```python
from build123d import *

# Parameters (mm, degrees)
F1_DEPTH = 45
F3_DEPTH = 45
F4_R     = 1.1
F5_DEPTH = 45
F6_R     = 3
F7_DEPTH = 0.1
F8_R     = 2.5
F9_DEPTH = 3


with BuildPart() as f1:
    # F0 (on Top) → F1 (new body)
    with BuildSketch(Plane.XY):
        with BuildLine():
            ThreePointArc((4.8636480497, -1.1597101572), (4.9657950143, -0.5838491892), (5, 0))
            ThreePointArc((5, 0), (4.9657950143, 0.5838491892), (4.8636480497, 1.1597101572))
            Line((4.8636480497, 1.1597101572), (1.294427191, 0))
            Line((1.294427191, 0), (4.8636480497, -1.1597101572))
        make_face()
        with BuildLine():
            Line((1.294427191, 0), (4.8636480497, 1.1597101572))
            ThreePointArc((4.8636480497, 1.1597101572), (4.7552825815, 1.5450849719), (4.6164344542, 1.9205553702))
            Line((4.6164344542, 1.9205553702), (1.0472135955, 0.760845213))
            Line((1.0472135955, 0.760845213), (0.6472135955, 0.2102924448))
            Line((0.6472135955, 0.2102924448), (1.294427191, 0))
        make_face()
        with BuildLine():
            ThreePointArc((4.6164344542, 1.9205553702), (4.7552825815, 1.5450849719), (4.8636480497, 1.1597101572))
            Line((4.8636480497, 1.1597101572), (67.6486194547, 21.5597839941))
            Line((67.6486194547, 21.5597839941), (67.4014058592, 22.3206292071))
            Line((67.4014058592, 22.3206292071), (4.6164344542, 1.9205553702))
        make_face()
        with BuildLine():
            Line((67.6486194547, -21.5597839941), (4.8636480497, -1.1597101572))
            ThreePointArc((4.8636480497, -1.1597101572), (4.7552825815, -1.5450849719), (4.6164344542, -1.9205553702))
            Line((4.6164344542, -1.9205553702), (67.4014058592, -22.3206292071))
            Line((67.4014058592, -22.3206292071), (67.6486194547, -21.5597839941))
        make_face()
        with BuildLine():
            ThreePointArc((4.6164344542, -1.9205553702), (4.7552825815, -1.5450849719), (4.8636480497, -1.1597101572))
            Line((4.8636480497, -1.1597101572), (1.294427191, 0))
            Line((1.294427191, 0), (0.6472135955, -0.2102924448))
            Line((0.6472135955, -0.2102924448), (1.0472135955, -0.760845213))
            Line((1.0472135955, -0.760845213), (4.6164344542, -1.9205553702))
        make_face()
        with BuildLine():
            Line((1.0472135955, 0.760845213), (4.6164344542, 1.9205553702))
            ThreePointArc((4.6164344542, 1.9205553702), (4.0450849719, 2.9389262615), (3.2531133995, 3.7970058217))
            Line((3.2531133995, 3.7970058217), (1.0472135955, 0.760845213))
        make_face()
        with BuildLine():
            ThreePointArc((3.2531133995, -3.7970058217), (4.0450849719, -2.9389262615), (4.6164344542, -1.9205553702))
            Line((4.6164344542, -1.9205553702), (1.0472135955, -0.760845213))
            Line((1.0472135955, -0.760845213), (3.2531133995, -3.7970058217))
        make_face()
        with BuildLine():
            Line((1.0472135955, 0.760845213), (3.2531133995, 3.7970058217))
            ThreePointArc((3.2531133995, 3.7970058217), (2.9389262615, 4.0450849719), (2.605899804, 4.2672340235))
            Line((2.605899804, 4.2672340235), (0.4, 1.2310734149))
            Line((0.4, 1.2310734149), (0.4, 0.5505527682))
            Line((0.4, 0.5505527682), (1.0472135955, 0.760845213))
        make_face()
        with BuildLine():
            ThreePointArc((2.605899804, 4.2672340235), (2.9389262615, 4.0450849719), (3.2531133995, 3.7970058217))
            Line((3.2531133995, 3.7970058217), (42.0563597105, 57.2050924997))
            Line((42.0563597105, 57.2050924997), (41.409146115, 57.6753207015))
            Line((41.409146115, 57.6753207015), (2.605899804, 4.2672340235))
        make_face()
        with BuildLine():
            Line((42.0563597105, -57.2050924997), (3.2531133995, -3.7970058217))
            ThreePointArc((3.2531133995, -3.7970058217), (2.9389262615, -4.0450849719), (2.605899804, -4.2672340235))
            Line((2.605899804, -4.2672340235), (41.409146115, -57.6753207015))
            Line((41.409146115, -57.6753207015), (42.0563597105, -57.2050924997))
        make_face()
        with BuildLine():
            ThreePointArc((2.605899804, -4.2672340235), (2.9389262615, -4.0450849719), (3.2531133995, -3.7970058217))
            Line((3.2531133995, -3.7970058217), (1.0472135955, -0.760845213))
            Line((1.0472135955, -0.760845213), (0.4, -0.5505527682))
            Line((0.4, -0.5505527682), (0.4, -1.2310734149))
            Line((0.4, -1.2310734149), (2.605899804, -4.2672340235))
        make_face()
        with BuildLine():
            Line((0.4, 1.2310734149), (2.605899804, 4.2672340235))
            ThreePointArc((2.605899804, 4.2672340235), (1.5450849719, 4.7552825815), (0.4, 4.9839743178))
            Line((0.4, 4.9839743178), (0.4, 1.2310734149))
        make_face()
        with BuildLine():
            ThreePointArc((0.4, -4.9839743178), (1.5450849719, -4.7552825815), (2.605899804, -4.2672340235))
            Line((2.605899804, -4.2672340235), (0.4, -1.2310734149))
            Line((0.4, -1.2310734149), (0.4, -4.9839743178))
        make_face()
        with BuildLine():
            Line((0.4, 1.2310734149), (0.4, 4.9839743178))
            ThreePointArc((0.4, 4.9839743178), (0, 5), (-0.4, 4.9839743178))
            Line((-0.4, 4.9839743178), (-0.4, 1.2310734149))
            Line((-0.4, 1.2310734149), (0, 0.6805206467))
            Line((0, 0.6805206467), (0.4, 1.2310734149))
        make_face()
        with BuildLine():
            ThreePointArc((-0.4, 4.9839743178), (0, 5), (0.4, 4.9839743178))
            Line((0.4, 4.9839743178), (0.4, 71))
            Line((0.4, 71), (-0.4, 71))
            Line((-0.4, 71), (-0.4, 4.9839743178))
        make_face()
        with BuildLine():
            Line((0.4, -71), (0.4, -4.9839743178))
            ThreePointArc((0.4, -4.9839743178), (0, -5), (-0.4, -4.9839743178))
            Line((-0.4, -4.9839743178), (-0.4, -71))
            Line((-0.4, -71), (0.4, -71))
        make_face()
        with BuildLine():
            ThreePointArc((-0.4, -4.9839743178), (0, -5), (0.4, -4.9839743178))
            Line((0.4, -4.9839743178), (0.4, -1.2310734149))
            Line((0.4, -1.2310734149), (0, -0.6805206467))
            Line((0, -0.6805206467), (-0.4, -1.2310734149))
            Line((-0.4, -1.2310734149), (-0.4, -4.9839743178))
        make_face()
        with BuildLine():
            Line((-0.4, 1.2310734149), (-0.4, 4.9839743178))
            ThreePointArc((-0.4, 4.9839743178), (-1.5450849719, 4.7552825815), (-2.605899804, 4.2672340235))
            Line((-2.605899804, 4.2672340235), (-0.4, 1.2310734149))
        make_face()
        with BuildLine():
            ThreePointArc((-2.605899804, -4.2672340235), (-1.5450849719, -4.7552825815), (-0.4, -4.9839743178))
            Line((-0.4, -4.9839743178), (-0.4, -1.2310734149))
            Line((-0.4, -1.2310734149), (-2.605899804, -4.2672340235))
        make_face()
        with BuildLine():
            Line((-0.4, 1.2310734149), (-2.605899804, 4.2672340235))
            ThreePointArc((-2.605899804, 4.2672340235), (-2.9389262615, 4.0450849719), (-3.2531133995, 3.7970058217))
            Line((-3.2531133995, 3.7970058217), (-1.0472135955, 0.760845213))
            Line((-1.0472135955, 0.760845213), (-0.4, 0.5505527682))
            Line((-0.4, 0.5505527682), (-0.4, 1.2310734149))
        make_face()
        with BuildLine():
            ThreePointArc((-3.2531133995, 3.7970058217), (-2.9389262615, 4.0450849719), (-2.605899804, 4.2672340235))
            Line((-2.605899804, 4.2672340235), (-41.409146115, 57.6753207015))
            Line((-41.409146115, 57.6753207015), (-42.0563597105, 57.2050924997))
            Line((-42.0563597105, 57.2050924997), (-3.2531133995, 3.7970058217))
        make_face()
        with BuildLine():
            Line((-41.409146115, -57.6753207015), (-2.605899804, -4.2672340235))
            ThreePointArc((-2.605899804, -4.2672340235), (-2.9389262615, -4.0450849719), (-3.2531133995, -3.7970058217))
            Line((-3.2531133995, -3.7970058217), (-42.0563597105, -57.2050924997))
            Line((-42.0563597105, -57.2050924997), (-41.409146115, -57.6753207015))
        make_face()
        with BuildLine():
            ThreePointArc((-3.2531133995, -3.7970058217), (-2.9389262615, -4.0450849719), (-2.605899804, -4.2672340235))
            Line((-2.605899804, -4.2672340235), (-0.4, -1.2310734149))
            Line((-0.4, -1.2310734149), (-0.4, -0.5505527682))
            Line((-0.4, -0.5505527682), (-1.0472135955, -0.760845213))
            Line((-1.0472135955, -0.760845213), (-3.2531133995, -3.7970058217))
        make_face()
        with BuildLine():
            Line((-1.0472135955, 0.760845213), (-3.2531133995, 3.7970058217))
            ThreePointArc((-3.2531133995, 3.7970058217), (-4.0450849719, 2.9389262615), (-4.6164344542, 1.9205553702))
            Line((-4.6164344542, 1.9205553702), (-1.0472135955, 0.760845213))
        make_face()
        with BuildLine():
            ThreePointArc((-4.6164344542, -1.9205553702), (-4.0450849719, -2.9389262615), (-3.2531133995, -3.7970058217))
            Line((-3.2531133995, -3.7970058217), (-1.0472135955, -0.760845213))
            Line((-1.0472135955, -0.760845213), (-4.6164344542, -1.9205553702))
        make_face()
        with BuildLine():
            Line((-1.0472135955, 0.760845213), (-4.6164344542, 1.9205553702))
            ThreePointArc((-4.6164344542, 1.9205553702), (-4.7552825815, 1.5450849719), (-4.8636480497, 1.1597101572))
            Line((-4.8636480497, 1.1597101572), (-1.294427191, 0))
            Line((-1.294427191, 0), (-0.6472135955, 0.2102924448))
            Line((-0.6472135955, 0.2102924448), (-1.0472135955, 0.760845213))
        make_face()
        with BuildLine():
            ThreePointArc((-4.8636480497, 1.1597101572), (-4.7552825815, 1.5450849719), (-4.6164344542, 1.9205553702))
            Line((-4.6164344542, 1.9205553702), (-67.4014058592, 22.3206292071))
            Line((-67.4014058592, 22.3206292071), (-67.6486194547, 21.5597839941))
            Line((-67.6486194547, 21.5597839941), (-4.8636480497, 1.1597101572))
        make_face()
        with BuildLine():
            Line((-67.4014058592, -22.3206292071), (-4.6164344542, -1.9205553702))
            ThreePointArc((-4.6164344542, -1.9205553702), (-4.7552825815, -1.5450849719), (-4.8636480497, -1.1597101572))
            Line((-4.8636480497, -1.1597101572), (-67.6486194547, -21.5597839941))
            Line((-67.6486194547, -21.5597839941), (-67.4014058592, -22.3206292071))
        make_face()
        with BuildLine():
            ThreePointArc((-4.8636480497, -1.1597101572), (-4.7552825815, -1.5450849719), (-4.6164344542, -1.9205553702))
            Line((-4.6164344542, -1.9205553702), (-1.0472135955, -0.760845213))
            Line((-1.0472135955, -0.760845213), (-0.6472135955, -0.2102924448))
            Line((-0.6472135955, -0.2102924448), (-1.294427191, 0))
            Line((-1.294427191, 0), (-4.8636480497, -1.1597101572))
        make_face()
        with BuildLine():
            Line((-1.294427191, 0), (-4.8636480497, 1.1597101572))
            ThreePointArc((-4.8636480497, 1.1597101572), (-5, 0), (-4.8636480497, -1.1597101572))
            Line((-4.8636480497, -1.1597101572), (-1.294427191, 0))
        make_face()
    extrude(amount=F1_DEPTH)

    # F2 (on face) → F3 (join)
    with BuildSketch(Plane(origin=(0, 0, 0), x_dir=(1, 0, 0), z_dir=(0, 0, -1))):
        Polygon((0.4, 1.2310734149), (0, 0.6805206467), (-0.4, 1.2310734149), (-0.4, 0.5505527682), (-1.0472135955, 0.760845213), (-0.6472135955, 0.2102924448), (-1.294427191, 0), (-0.6472135955, -0.2102924448), (-1.0472135955, -0.760845213), (-0.4, -0.5505527682), (-0.4, -1.2310734149), (0, -0.6805206467), (0.4, -1.2310734149), (0.4, -0.5505527682), (1.0472135955, -0.760845213), (0.6472135955, -0.2102924448), (1.294427191, 0), (0.6472135955, 0.2102924448), (1.0472135955, 0.760845213), (0.4, 0.5505527682), align=None)
    extrude(amount=-F3_DEPTH)

    # F4 (on face) → F5 (cut, through all)
    with BuildSketch(Plane.XY.offset(45)):
        Circle(F4_R)
    extrude(amount=-F5_DEPTH, mode=Mode.SUBTRACT)

    # F6 (on face) → F7 (cut)
    with BuildSketch(Plane.XY.offset(45)):
        Circle(F6_R)
    extrude(amount=-F7_DEPTH, mode=Mode.SUBTRACT)

    # F8 (on face) → F9 (cut)
    with BuildSketch(Plane.XY.offset(44.9)):
        Circle(F8_R)
    extrude(amount=-F9_DEPTH, mode=Mode.SUBTRACT)


solid = f1.part
```
Model file for the job. Use its own axes, mm. A direction names the side the tool comes from. Give positions to 0.01 mm unless a question says otherwise; leave off trailing zeros. Loops run counter-clockwise (first coordinate to the right, second up) from the corner with the lowest first, then second, coordinate; pieces in that order, holes last. Notation, with made-up numbers: (-4, 87) -> (11, 87) arc R24 cw to (11, 105) -> close; hole circle Ø10 at (87.5, 49). An arc over 180 degrees is marked (long way). Use CSV: the item, a comma, the result in double quotes. Start each with the question number.
1) Wall check: line 1 (Y direction, x = 0, z = 31.5); line 2 (X direction, y = 26, z = 8.5); line 3 (Y direction, x = 0, z = 44.95). Give the ranges that are in metal, low to high.
2) Mould opens along X. For faces 1 (the flat face through (36.696, -11.503, 22.185)), 2 (the flat face through (0, -6, 0)), 3 (the flat face through (21.74, -30.6, 22.18)) say: released by +X, released by -X, zero draft, split by the parting line, or undercut.
3) Tool access for faces 4 (the cylindrical face through (-0.54, -2.44, 43.42)), 5 (the flat face through (-21.74, 30.6, 22.18)), 6 (the flat face through (0.4, -38, 22)), 7 (the flat face through (36.448, 12.263, 22.185)): list every direction of +Z, -Z, +X, -X, +Y, -Y with a clear straight run to the whole face (end or side of a thin tool).
4) Slice it at B-B on x = -27. Give the cut face in (y, z).
5) Flat gauge pins, fed straight in: pin 1 Ø4 at (x, z) = (6, 32) entering from +Y; pin 2 Ø22.5 at (y, z) = (-43, 30) entering from +X; pin 3 Ø2 at (x, z) = (-32, 36) entering from +Y. Where does each tip first touch, or does it go through?
6) Slice it at A-A on y = 31. Give the cut face in (x, z).
7) Slice it at C-C on y = 15.5. Give the cut face in (x, z), plus the area to 3 significant figures.
Computed values:
1,line 1,"y = -71 to -1.1, 1.1 to 71"
1,line 2,"x = -19.38 to -18.4, -0.4 to 0.4, 18.4 to 19.38"
1,line 3,"y = -71 to -3, 3 to 71"
2,face 1,"released by +X"
2,face 2,"zero draft"
2,face 3,"undercut"
3,face 4,"+Z"
3,face 5,"+Z, -Z, +Y"
3,face 6,"+Z, -Z, -Y"
3,face 7,"+Z, -Z"
4,outline,"(-37.84, 0) -> (-36.48, 0) -> (-36.48, 45) -> (-37.84, 45) -> close; (-9.19, 0) -> (-8.35, 0) -> (-8.35, 45) -> (-9.19, 45) -> close; (8.35, 0) -> (9.19, 0) -> (9.19, 45) -> (8.35, 45) -> close; (36.48, 0) -> (37.84, 0) -> (37.84, 45) -> (36.48, 45) -> close"
5,pin 1,"stops at y = 11.69"
5,pin 2,"stops at x = 39.91"
5,pin 3,"stops at y = 46.1"
6,outline,"(-23.02, 0) -> (-22.03, 0) -> (-22.03, 45) -> (-23.02, 45) -> close; (-0.4, 0) -> (0.4, 0) -> (0.4, 45) -> (-0.4, 45) -> close; (22.03, 0) -> (23.02, 0) -> (23.02, 45) -> (22.03, 45) -> close"
7,outline,"(-49, 0) -> (-46.41, 0) -> (-46.41, 45) -> (-49, 45) -> close; (-11.76, 0) -> (-10.77, 0) -> (-10.77, 45) -> (-11.76, 45) -> close; (-0.4, 0) -> (0.4, 0) -> (0.4, 45) -> (-0.4, 45) -> close; (10.77, 0) -> (11.76, 0) -> (11.76, 45) -> (10.77, 45) -> close; (46.41, 0) -> (49, 0) -> (49, 45) -> (46.41, 45) -> close"
7,area,"358 mm^2"
